Study the drawing (mm; zero at the part's minimum x, y, z) and answer. A direction names the side the tool comes from. Give positions to 0.01 mm unless a question says otherwise; leave off trailing zeros. Write each loop counter-clockwise with the first axis right and the second up, starting at its lowest first coordinate (ties: lowest second). Pieces come first, ordered by that corner, then holes. Notation, with made-up numbers: M 6,65 L 49,65 A19 cw 49,102 Z; hole C 78,45 d3. An arc over 180 degrees is marked long. Use a Markdown table: item, result. Add a question column.
Item 1: A cutting plane is placed at A-A on y = 1.25. Determine the outline of the cut face in (x, z) (3 decimals).
Item 2: Consider probe 1 along Z at (x, y) = (0.7, 2.25); probe 2 along Y at (x, z) = (0.85, 21.75) (3 decimals); probe 3 along X at (y, z) = (0.6, 18.5). Determine where each line is inside the solid, lowest interval first. Write a range as [from, to].
Item 3: A cutting plane is placed at B-B on x = 1.15. Determine the outline of the cut face in (y, z) (3 decimals).
Item 4: For the marked faces 1, 2 and 3, determine the directions among +Z, -Z, +X, -X, +Y, -Y from which every point of the face is accessible in a straight line to the end or side of a thin tool.
Item 5: Given P1, Ø0.9, axis at x = 1, z = 22.5, coming from the +Y side (3 decimals); P2, Ø0.5, axis at y = 1, z = 23.5, coming from the -X side (3 decimals); P3, Ø0.5, axis at x = 1, z = 24, coming from the -Y side (3 decimals), each flat-ended and moving along its own axis, determine where each tip first touches the part or whether it passes through.
Item 6: A cutting plane is placed at C-C on z = 20.75. Determine the outline of the cut face in (x, y) (3 decimals), then the cut area to 3 significant figures.
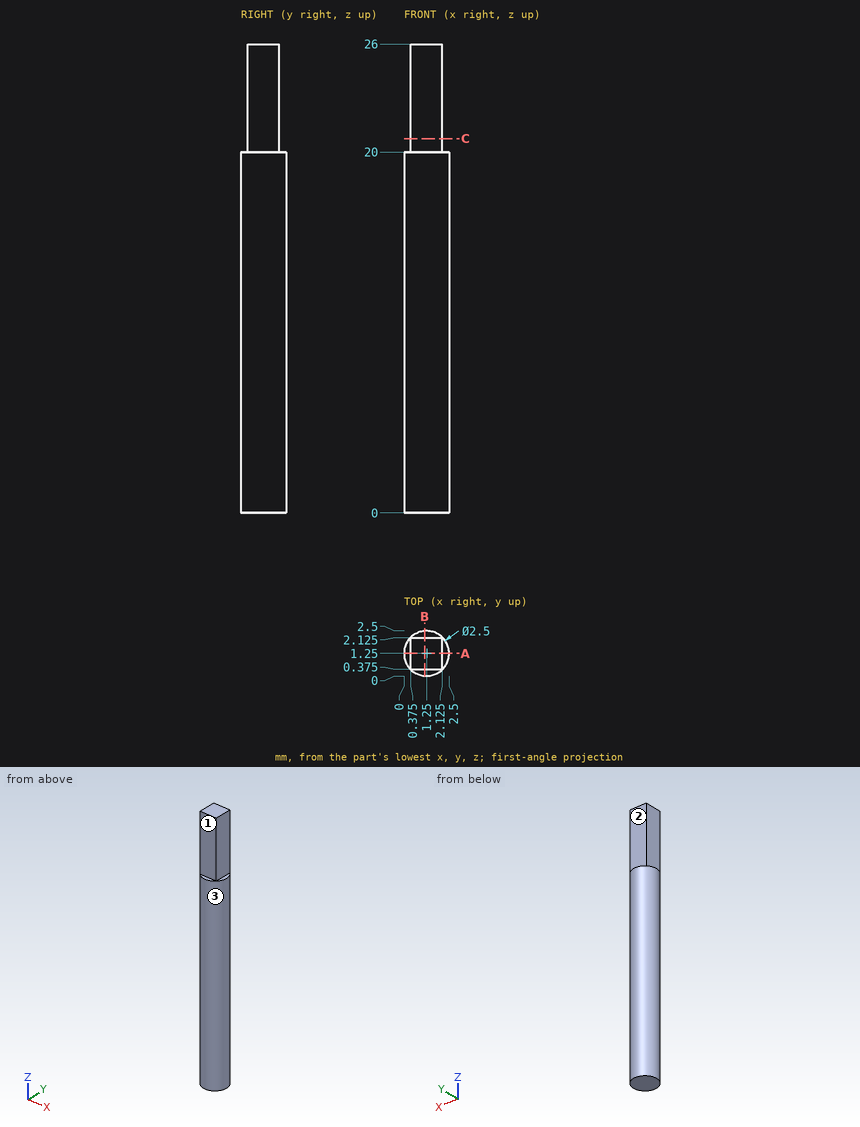
Filled in:
| question | item | result |
|---|---|---|
| 1 | outline | M 0,0 L 2.5,0 L 2.5,20 L 2.125,20 L 2.125,26 L 0.375,26 L 0.375,20 L 0,20 Z |
| 2 | probe 1 | [0, 20] |
| 2 | probe 2 | [0.375, 2.125] |
| 2 | probe 3 | [0.18, 2.32] |
| 3 | outline | M 0.004,0 L 2.496,0 L 2.496,20 L 2.125,20 L 2.125,26 L 0.375,26 L 0.375,20 L 0.004,20 Z |
| 4 | face 1 | +Z, +X, -X, -Y |
| 4 | face 2 | +Z, +X, -X, +Y |
| 4 | face 3 | +Z, -Z |
| 5 | P1 | y = 2.125 |
| 5 | P2 | x = 0.375 |
| 5 | P3 | y = 0.375 |
| 6 | outline | M 0.375,0.375 L 2.125,0.375 L 2.125,2.125 L 0.375,2.125 Z |
| 6 | area | 3.06 mm² |
